Geometry: see drawing. Coordinates: mm, zero at the bounding-box minimum. A direction names the side the tool comes from. Round coordinates to 2 decimals unless told otherwise and drop trailing zeros. Order: outer loops, then holes, each group sorted by start corner. A loop starts at its lowest first (then second) coordinate and runs counter-clockwise, first axis right, second up. Notation, with made-up numbers: (43, -9) -> (61, -9) arc R16 ccw to (61, -5) -> close; hole circle Ø4 at (28, 80.5). An arc over 180 degrees is marked (long way). Put each result on its own line as item: value.
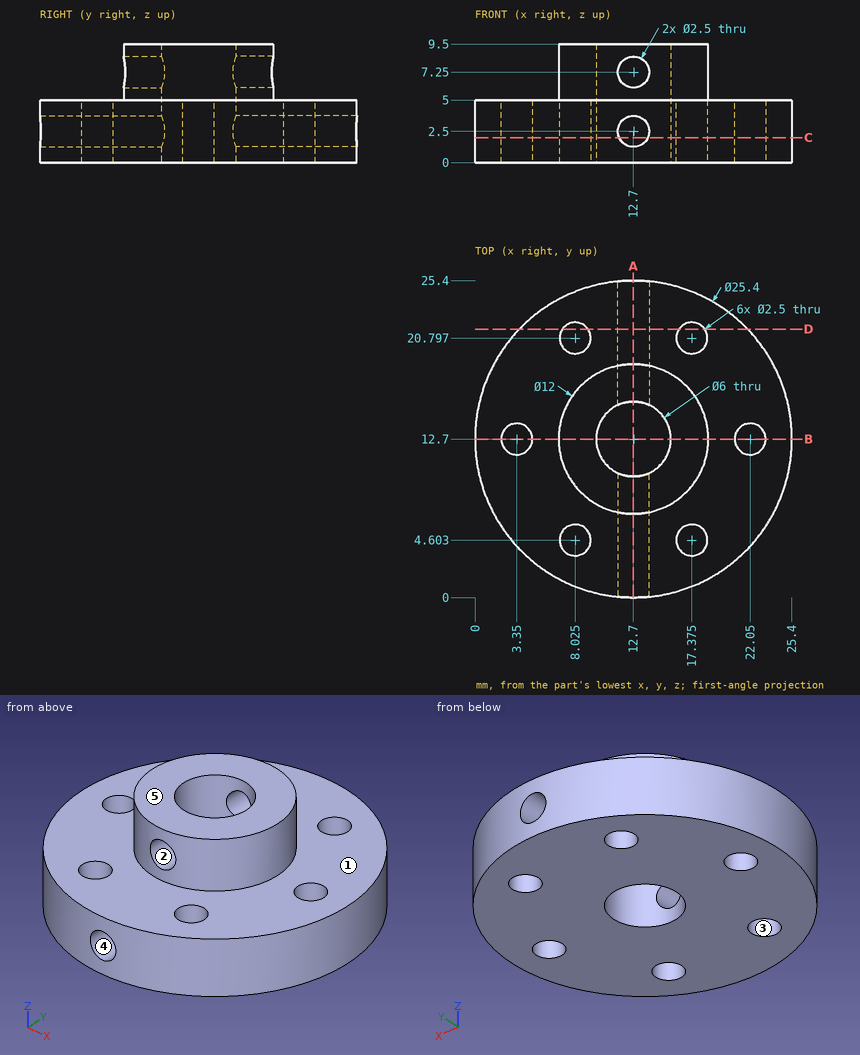
1. Material intervals for probe 1 along X at (y, z) = (5.5, 2) (1 decimal); probe 2 along X at (y, z) = (12.5, 6); probe 3 along X at (y, z) = (21, 3) (1 decimal), sorted ascending.
Ans:
probe 1: 2.2 to 7.2, 8.9 to 11.6, 13.8 to 16.5, 18.2 to 23.2
probe 2: 6.7 to 9.71, 15.69 to 18.7
probe 3: 3.1 to 6.8, 9.3 to 11.6, 13.8 to 16.1, 18.6 to 22.3
2. Cut plane B-B on y = 12.7. Return loops of the section in (x, z).
Ans:
outline: (0, 0) -> (2.1, 0) -> (2.1, 5) -> (0, 5) -> close; (4.6, 0) -> (9.7, 0) -> (9.7, 9.5) -> (6.7, 9.5) -> (6.7, 5) -> (4.6, 5) -> close; (15.7, 0) -> (20.8, 0) -> (20.8, 5) -> (18.7, 5) -> (18.7, 9.5) -> (15.7, 9.5) -> close; (23.3, 0) -> (25.4, 0) -> (25.4, 5) -> (23.3, 5) -> close
3. Cut plane A-A on x = 12.7. Return loops of the section in (y, z).
Ans:
outline: (0, 0) -> (9.7, 0) -> (9.7, 1.25) -> (0, 1.25) -> close; (0, 3.75) -> (9.7, 3.75) -> (9.7, 6) -> (6.7, 6) -> (6.7, 5) -> (0, 5) -> close; (6.7, 8.5) -> (9.7, 8.5) -> (9.7, 9.5) -> (6.7, 9.5) -> close; (15.7, 0) -> (25.4, 0) -> (25.4, 1.25) -> (15.7, 1.25) -> close; (15.7, 3.75) -> (25.4, 3.75) -> (25.4, 5) -> (18.7, 5) -> (18.7, 6) -> (15.7, 6) -> close; (15.7, 8.5) -> (18.7, 8.5) -> (18.7, 9.5) -> (15.7, 9.5) -> close
4. Contact query for flat-ended pins moving along their axis: P1, Ø3, axis at x = 12.7, z = 7.25, coming from the -Y side; P2, Ø4, axis at x = 3.35, y = 12.7, coming from the +Z side; P3, Ø5, axis at y = 16, z = 2.5, coming from the -X side (1 decimal). Output: stop coordinate, or through.
Ans:
P1: y = 6.7
P2: z = 5
P3: x = 0
5. Cut plane D-D on y = 21.5. Return loops of the section in (x, z).
Ans:
outline: (3.54, 0) -> (6.99, 0) -> (6.99, 5) -> (3.54, 5) -> close; (9.06, 0) -> (16.34, 0) -> (16.34, 5) -> (9.06, 5) -> close; (18.41, 0) -> (21.86, 0) -> (21.86, 5) -> (18.41, 5) -> close; hole circle Ø2.5 at (12.7, 2.5)
6. Draft query along Z for the marked faces 3, 4 and 5. Return one class per face: +Z half, -Z half, draft (parallel to the pull), parting line (faces both ways), or undercut.
Ans:
face 3: draft
face 4: undercut
face 5: +Z half
7. Set-up query: the marked faces 1 and 2. Return all of +Z, -Z, +X, -X, +Y, -Y with unobstructed straight access to the full face (end or side cutting, diameter ignored); none if empty.
Ans:
face 1: +Z
face 2: +Y, -Y
8. Cut plane C-C on z = 2. State how many separate pieces and enclosed holes the cut face has, and give its area (3 significant figures).
Ans:
separate pieces: 2
enclosed holes: 6
area: 404 mm²
